from build123d import *

# Parameters (mm, degrees)
BOSS_EXTRUDE1_START = 65
SKETCH1_W           = 135
SKETCH1_H           = 115.198794821
BOSS_EXTRUDE1_DEPTH = 8
SKETCH2_W           = 10
SKETCH2_H           = 5
CUT_EXTRUDE1_DEPTH  = 9
SKETCH3_R           = 1.25
CUT_EXTRUDE2_DEPTH  = 9
CHAMFER2_SIZE       = 1


with BuildPart() as part:
    # Sketch1 → Boss-Extrude1 (new body)
    with BuildSketch(Plane.XY.offset(BOSS_EXTRUDE1_START)):
        with Locations((0, 37.599397411)):
            Rectangle(SKETCH1_W, SKETCH1_H)
    extrude(amount=BOSS_EXTRUDE1_DEPTH)

    # Sketch2 → Cut-Extrude1 (cut, through all)
    with BuildSketch(Plane.XY.offset(73)):
        with Locations((-40.5, 45.346)):
            Rectangle(SKETCH2_W, SKETCH2_H)
    extrude(amount=-CUT_EXTRUDE1_DEPTH, mode=Mode.SUBTRACT)

    # Sketch3 → Cut-Extrude2 (cut, through all)
    with BuildSketch(Plane.XY.offset(73)):
        with Locations((-21.5, 72.116)):
            Circle(SKETCH3_R)
        with Locations((-49.5, 44.176)):
            Circle(SKETCH3_R)
    extrude(amount=-CUT_EXTRUDE2_DEPTH, mode=Mode.SUBTRACT)

    # Chamfer2
    chamfer2_edges = [part.edges().sort_by_distance(p)[0] for p in [
        (-40.5, 47.846, 73),
        (-45.5, 45.346, 73),
        (-40.5, 42.846, 73),
        (-35.5, 45.346, 73),
    ]]
    chamfer(chamfer2_edges, length=CHAMFER2_SIZE)


solid = part.part
Can you work these out from the model? Positions are in its coordinate system, mm. A direction names the side the tool comes from. Round coordinates to 2 decimals unless told otherwise and drop trailing zeros. Use one line per item in the form item = value. Start each with the question number.
Q1. We'd pull the mould along Y, two halves only. Please class faces 3 (the face through (-1, 38, 65)), 4 (the face through (-45.5, 45, 69)), 5 (the face through (-1, -20, 69)): +Y half, -Y half, draft (parallel to the pull), parting line (faces both ways), or undercut.
Q2. If I drill on probe 1 along Y at (x, z) = (-49.5, 70.5); probe 2 along Y at (x, z) = (-21.5, 66.5), over which ranges is the centre line in solid material (lowest first)? Write a range as [from, to].
Q3. Which directions (+Z, -Z, +X, -X, +Y, -Y) give clear straight access to the entire face, cutting with the end or side of a thin tool? Please do faces 1 (the face through (-41, 47.846, 69)), 2 (the face through (-1, 95.199, 69)).
Worked out:
q1.face_3 = draft
q1.face_4 = undercut
q1.face_5 = -Y half
q2.probe_1 = [-20, 42.93], [45.43, 95.2]
q2.probe_2 = [-20, 70.87], [73.37, 95.2]
q3.face_1 = +Z, -Z
q3.face_2 = +Z, -Z, +X, -X, +Y
